from build123d import *

# Parameters (mm, degrees)
SKETCH1_W           = 23
SKETCH1_H           = 74
SKETCH1_R           = 1.5
BOSS_EXTRUDE1_DEPTH = 2
SKETCH1_3_W         = 2
SKETCH1_3_H         = 74
BOSS_EXTRUDE2_DEPTH = 45
FILLET1_R           = 1
FILLET2_R           = 20
SKETCH2_R           = 5
CUT_EXTRUDE1_DEPTH  = 2


with BuildPart() as part:
    # Sketch1 → Boss-Extrude1 (new body)
    with BuildSketch(Plane(origin=(0, 0, 0), x_dir=(1, 0, 0), z_dir=(0, 1, 0))):
        with Locations((13.5, 37)):
            Rectangle(SKETCH1_W, SKETCH1_H)
        with Locations((7.25, 7)):
            Circle(SKETCH1_R, mode=Mode.SUBTRACT)
        with Locations((17.75, 7)):
            Circle(SKETCH1_R, mode=Mode.SUBTRACT)
        with Locations((7.25, 67)):
            Circle(SKETCH1_R, mode=Mode.SUBTRACT)
        with Locations((17.75, 67)):
            Circle(SKETCH1_R, mode=Mode.SUBTRACT)
    extrude(amount=BOSS_EXTRUDE1_DEPTH)

    # Sketch1<3> → Boss-Extrude2 (add)
    with BuildSketch(Plane(origin=(0, 0, 0), x_dir=(1, 0, 0), z_dir=(0, 1, 0))):
        with Locations((1, 37)):
            Rectangle(SKETCH1_3_W, SKETCH1_3_H)
    extrude(amount=BOSS_EXTRUDE2_DEPTH)

    # Fillet1
    fillet1_edges = [part.edges().sort_by_distance(p)[0] for p in [
        (0, 0, -37),
        (2, 2, -37),
    ]]
    fillet(fillet1_edges, radius=FILLET1_R)

    # Fillet2
    fillet2_edges = [part.edges().sort_by_distance(p)[0] for p in [
        (1, 45, -74),
        (1, 45, 0),
    ]]
    fillet(fillet2_edges, radius=FILLET2_R)

    # Sketch2 → Cut-Extrude1 (cut)
    with BuildSketch(Plane.ZY):
        with Locations((-37, 30)):
            Circle(SKETCH2_R)
    extrude(amount=-CUT_EXTRUDE1_DEPTH, mode=Mode.SUBTRACT)


solid = part.part
Geometry: final body of the model. Coordinates: model frame, mm. A direction names the side the tool comes from. Round coordinates to 2 decimals unless told otherwise and drop trailing zeros. Loops run counter-clockwise (first coordinate to the right, second up) from the corner with the lowest first, then second, coordinate; pieces in that order, holes last. Notation, with made-up numbers: M 50.25,-37 L 89.25,-37 A26 cw 89.25,-3 Z; hole C 22,40 d1. An arc over 180 degrees is marked long. Put each result on its own line as item: value. Start each with the question number.
(1) Section query A-A (x = 7.25). Return loops of the section in (y, z), then the cut area to 3 significant figures.
(2) Set-up query: faces 5 (the face through (14, 2, -38)), 6 (the face through (7.055, 0.986, -68.487)). Return all of +Z, -Z, +X, -X, +Y, -Y with unobstructed straight access to the full face (end or side cutting, diameter ignored); none if empty.
(3) Section query C-C (z = -51.5). Return loops of the section in (x, y).
(4) Draft query along Z for faces 1 (the face through (2, 24, -36)), 2 (the face through (16.25, 0.99, -7.07)), 3 (the face through (1, 30, -42)), 4 (the face through (1, 7, 0)). Return one class per face: +Z half, -Z half, draft (parallel to the pull), parting line (faces both ways), or undercut.
(5) Section query B-B (y = 30). Return loops of the section in (x, z), then the cut area to 3 significant figures.
(6) Contact query for flat-ended pins moving along their axis: pin 1 Ø1 at (y, z) = (22.5, -26) entering from +X; pin 2 Ø3.5 at (x, z) = (7.25, -7) entering from +Y; pin 3 Ø1.8 at (x, z) = (7.25, -67) entering from -Y. Output: stop coordinate, or through.
(7) Section query D-D (z = -7). Return loops of the section in (x, y).
(8) Material intervals for line 1 along Z through (x, y) = (7.25, 0.7); line 2 along X through (y, z) = (1, -7); line 3 along X through (y, z) = (5, -29.5), sorted ascending. Write a range as [from, to].
Findings below:
1. outline: M 0,-74 L 2,-74 L 2,-68.5 L 0,-68.5 Z; M 0,-65.5 L 2,-65.5 L 2,-8.5 L 0,-8.5 Z; M 0,-5.5 L 2,-5.5 L 2,0 L 0,0 Z
1. area: 136 mm2
2. face 5: +Z, -Z, +X, +Y
2. face 6: +Y, -Y
3. outline: M 0,1 A1 ccw 1,0 L 25,0 L 25,2 L 3,2 A1 cw 2,3 L 2,45 L 0,45 Z
4. face 1: draft
4. face 2: undercut
4. face 3: undercut
4. face 4: +Z half
5. outline: M 0,-73.36 L 2,-73.36 L 2,-42 L 0,-42 Z; M 0,-32 L 2,-32 L 2,-0.64 L 0,-0.64 Z
5. area: 125 mm2
6. pin 1: stops at x = 2
6. pin 2: stops at y = 2
6. pin 3: passes through
7. outline: M 0,1 A1 ccw 1,0 L 5.75,0 L 5.75,2 L 3,2 A1 cw 2,3 L 2,40.2 L 0,40.2 Z; M 8.75,0 L 16.25,0 L 16.25,2 L 8.75,2 Z; M 19.25,0 L 25,0 L 25,2 L 19.25,2 Z
8. line 1: z = [-74, -68.5], [-65.5, -8.5], [-5.5, 0]
8. line 2: x = [0, 5.75], [8.75, 16.25], [19.25, 25]
8. line 3: x = [0, 2]
